Could you check a few things on this model? Use its own coordinates, in mm. Give positions to 0.01 mm unless a question says otherwise; leave off trailing zeros. Order: outer loops, then holes, each group sorted by start corner. A loop starts at its lowest first (then second) coordinate and runs counter-clockwise, first axis right, second up.
(1) Imagine slicing it at D-D, the plane z = -27. Write out the boundary of the cut face in (x, y) (3 decimals).
(2) If we mould it in two halves opening along Z, with no side actions, what happens to faces 1 (the cylindrical face through (53.733, 1.565, -50.108)), 2 (the cylindrical face through (121.651, 1.565, -7.047)), 3 (the flat face through (97.025, 1.565, -66.639))? For each: released by +Z, released by -Z, zero draft, split by the parting line, or undercut.
(3) Imagine slicing it at A-A, the plane x = 53.5. Write out the boundary of the cut face in (y, z) (3 decimals).
(4) Imagine slicing it at B-B, the plane y = 2.2. Write out the boundary of the cut face in (x, z), then the cut area to 3 significant figures.
(5) Imagine slicing it at C-C, the plane z = -98.5. Write out the boundary of the cut face in (x, y) (3 decimals).
(6) If I drill on probe 1 along Z at (x, y) = (56, 1.3); probe 2 along X at (y, z) = (2.9, -19.5); probe 3 along Z at (x, y) = (102.5, 2.05), over which ranges is the centre line in solid material (lowest first)?
from build123d import *

# Parameters (mm, degrees)
SKETCH1_R           = 3.96875
SKETCH1_R_2         = 6.35
BOSS_EXTRUDE1_DEPTH = 3.175


with BuildPart() as part:
    # Sketch1 → Boss-Extrude1 (new body)
    with BuildSketch(Plane(origin=(0, 0, 0), x_dir=(1, 0, 0), z_dir=(0, 1, 0))):
        with BuildLine():
            Line((0, 0), (109.1184, 0))
            ThreePointArc((109.1184, 0), (121.760823269, 7.229815564), (121.940842268, 21.792394057))
            Line((121.940842268, 21.792394057), (71.401285641, 112.759573229))
            ThreePointArc((71.401285641, 112.759573229), (56.609708232, 121.4628), (41.818130824, 112.759573229))
            Line((41.818130824, 112.759573229), (-10.713122761, 18.207498065))
            ThreePointArc((-10.713122761, 18.207498065), (-10.562717277, 6.040495255), (0, 0))
        make_face()
        with Locations((5.658509088, 16.357983524)):
            Circle(SKETCH1_R, mode=Mode.SUBTRACT)
        with Locations((102.076909088, 16.357983524)):
            Circle(SKETCH1_R, mode=Mode.SUBTRACT)
        with Locations((54.5592, 100.77924387)):
            Circle(SKETCH1_R, mode=Mode.SUBTRACT)
        with Locations((54.5592, 43.812190688)):
            Circle(SKETCH1_R_2, mode=Mode.SUBTRACT)
    extrude(amount=BOSS_EXTRUDE1_DEPTH)


solid = part.part
Answer block:
1. outline: (-5.828, 0) - (119.048, 0) - (119.048, 3.175) - (-5.828, 3.175) - close
2. face 1: undercut
2. face 2: split by the parting line
2. face 3: released by -Z
3. outline: (0, -121.175) - (3.175, -121.175) - (3.175, -104.604) - (0, -104.604) - close; (0, -96.954) - (3.175, -96.954) - (3.175, -50.073) - (0, -50.073) - close; (0, -37.551) - (3.175, -37.551) - (3.175, 0) - (0, 0) - close
4. outline: (-10.71, -18.21) - (41.82, -112.76) arc R16.92 ccw to (71.4, -112.76) - (121.94, -21.79) arc R14.67 ccw to (109.12, 0) - (0, 0) arc R12.26 ccw to start; hole circle Ø7.94 at (5.66, -16.36); hole circle Ø12.7 at (54.56, -43.81); hole circle Ø7.94 at (54.56, -100.78); hole circle Ø7.94 at (102.08, -16.36)
4. area: 10,100 mm2
5. outline: (33.896, 0) - (51.31, 0) - (51.31, 3.175) - (33.896, 3.175) - close; (57.808, 0) - (79.324, 0) - (79.324, 3.175) - (57.808, 3.175) - close
6. probe 1: z = -121.45 to -104.48, -97.08 to -50, -37.63 to 0
6. probe 2: x = -10 to 3.23, 8.08 to 99.65, 104.5 to 122.97
6. probe 3: z = -56.78 to -20.3, -12.41 to 0
